Geometry check sheet. Reference: the model listing, model coordinates, mm. Round coordinates to 2 decimals unless told otherwise and drop trailing zeros. Use a Markdown table: item, result. Add a question column.
(1) Gauge pin test, flat ends, axial feed: P1, Ø17, axis at x = 3.27, z = 51.04, coming from the +Y side; P2, Ø4.5, axis at x = -8.04, z = -37.64, coming from the -Y side. Record the tip position at first contact, or that the pin passes through.
(2) Mould release check, pull along X, two halves, no side actions. Record for faces 1 (the face through (-9, 2, 71.041)), 2 (the face through (-8.64, 1.98, 37.82)), 3 (the face through (21.272, 2, 2)): released by +X, released by -X, zero draft, split by the parting line, or undercut.
(3) Section check A-A on y = 1.75. Give the number of separate pieces and of enclosed holes in the cut face, then the cut area to 3 significant figures.
(4) Thickness scan on line 1 along X through (y, z) = (3.25, -49); line 2 along X through (y, z) = (2.55, 38); line 3 along Z through (x, y) = (-2.5, 0.4). Record the ranges inside material, lowest first. Write a range as [from, to].
```python
from build123d import *

# Parameters (mm, degrees)
CROQUIS1_W              = 60
CROQUIS1_H              = 140
CROQUIS1_R              = 2
CROQUIS1_R_2            = 5
CROQUIS1_R_3            = 10.5
CROQUIS1_R_4            = 1.5
SALIENTE_EXTRUIR1_DEPTH = 4
CHAFL_N1_SIZE           = 0.5


with BuildPart() as part:
    # Croquis1 → Saliente-Extruir1 (new body)
    with BuildSketch(Plane(origin=(0, 0, 0), x_dir=(1, 0, 0), z_dir=(0, 1, 0))):
        with Locations((-8.728313692, -1.041413592)):
            Rectangle(CROQUIS1_W, CROQUIS1_H)
        with Locations(Location((3.271686308, 6.958586408, 0), (0, 0, 270))):
            Circle(CROQUIS1_R, mode=Mode.SUBTRACT)
        with Locations(Location((3.271686308, -9.041413592, 0), (0, 0, 270))):
            Circle(CROQUIS1_R, mode=Mode.SUBTRACT)
        with Locations(Location((14.585394807, 60.272294907, 0), (0, 0, 270))):
            Circle(CROQUIS1_R, mode=Mode.SUBTRACT)
        with Locations(Location((14.585394807, -39.727705093, 0), (0, 0, 270))):
            Circle(CROQUIS1_R, mode=Mode.SUBTRACT)
        with Locations(Location((-8.042022191, -39.727705093, 0), (0, 0, 90))):
            Circle(CROQUIS1_R, mode=Mode.SUBTRACT)
        with Locations(Location((-8.042022191, -62.355122091, 0), (0, 0, 270))):
            Circle(CROQUIS1_R, mode=Mode.SUBTRACT)
        with Locations(Location((3.271686308, -1.041413592, 0), (0, 0, 270))):
            Circle(CROQUIS1_R_2, mode=Mode.SUBTRACT)
        with Locations(Location((14.585394807, -62.355122091, 0), (0, 0, 90))):
            Circle(CROQUIS1_R, mode=Mode.SUBTRACT)
        with Locations(Location((3.271686308, -51.041413592, 0), (0, 0, 270))):
            Circle(CROQUIS1_R_3, mode=Mode.SUBTRACT)
        with Locations(Location((3.271686308, 48.958586408, 0), (0, 0, 270))):
            Circle(CROQUIS1_R_3, mode=Mode.SUBTRACT)
        with Locations(Location((-8.042022191, 60.272294907, 0), (0, 0, 90))):
            Circle(CROQUIS1_R, mode=Mode.SUBTRACT)
        with Locations(Location((14.585394807, 37.644877909, 0), (0, 0, 90))):
            Circle(CROQUIS1_R, mode=Mode.SUBTRACT)
        with Locations(Location((-8.042022191, 37.644877909, 0), (0, 0, 270))):
            Circle(CROQUIS1_R, mode=Mode.SUBTRACT)
        with Locations(Location((-21.728313692, -51.041413592, 0), (0, 0, 270))):
            Circle(CROQUIS1_R_4, mode=Mode.SUBTRACT)
        with Locations(Location((-33.728313692, -51.041413592, 0), (0, 0, 270))):
            Circle(CROQUIS1_R_4, mode=Mode.SUBTRACT)
        with Locations(Location((-21.728313692, 48.958586408, 0), (0, 0, 90))):
            Circle(CROQUIS1_R_4, mode=Mode.SUBTRACT)
        with Locations(Location((-33.728313692, 48.958586408, 0), (0, 0, 90))):
            Circle(CROQUIS1_R_4, mode=Mode.SUBTRACT)
    extrude(amount=SALIENTE_EXTRUIR1_DEPTH)

    # Chaflán1
    chafl_n1_edges = [part.edges().sort_by_distance(p)[0] for p in [
        (21.271686308, 4, 1.041413592),
        (3.271686308, 0, -8.958586408),
        (3.271686308, 4, -8.958586408),
        (-8.728313692, 4, -68.958586408),
        (3.271686308, 0, 7.041413592),
        (3.271686308, 4, 7.041413592),
        (14.585394807, 0, 37.727705093),
        (14.585394807, 4, 37.727705093),
        (-8.042022191, 0, 41.727705093),
        (-8.042022191, 4, 41.727705093),
        (3.271686308, 0, -3.958586408),
        (3.271686308, 4, -3.958586408),
        (-8.042022191, 0, 60.355122091),
        (-8.042022191, 4, 60.355122091),
        (3.271686308, 0, 40.541413592),
        (3.271686308, 4, 40.541413592),
        (3.271686308, 0, -59.458586408),
        (3.271686308, 4, -59.458586408),
        (-38.728313692, 4, 1.041413592),
        (14.585394807, 0, 64.355122091),
        (14.585394807, 4, 64.355122091),
        (-8.728313692, 0, -68.958586408),
        (14.585394807, 0, -62.272294907),
        (14.585394807, 4, -62.272294907),
        (21.271686308, 0, 1.041413592),
        (-8.042022191, 0, -58.272294907),
        (-8.042022191, 4, -58.272294907),
        (-8.728313692, 0, 71.041413592),
        (14.585394807, 0, -35.644877909),
        (14.585394807, 4, -35.644877909),
        (-38.728313692, 0, 1.041413592),
        (-8.042022191, 0, -39.644877909),
        (-8.042022191, 4, -39.644877909),
        (-21.728313692, 0, 49.541413592),
        (-21.728313692, 4, 49.541413592),
        (-33.728313692, 0, 49.541413592),
        (-33.728313692, 4, 49.541413592),
        (-21.728313692, 0, -47.458586408),
        (-21.728313692, 4, -47.458586408),
        (-8.728313692, 4, 71.041413592),
        (-33.728313692, 0, -47.458586408),
        (-33.728313692, 4, -47.458586408),
        (-38.728313692, 2, -68.958586408),
        (21.271686308, 2, -68.958586408),
        (21.271686308, 2, 71.041413592),
        (-38.728313692, 2, 71.041413592),
    ]]
    chamfer(chafl_n1_edges, length=CHAFL_N1_SIZE - 0.0001)  # a hair under: the kernel refuses the full size


solid = part.part
```
Check sheet entries:
| question | item | result |
|---|---|---|
| 1 | P1 | passes through |
| 1 | P2 | stops at y = 0.24 |
| 2 | face 1 | zero draft |
| 2 | face 2 | undercut |
| 2 | face 3 | released by +X |
| 3 | separate pieces | 1 |
| 3 | enclosed holes | 17 |
| 3 | area | 7,470 mm2 |
| 4 | line 1 | x = [-38.73, -35.23], [-32.23, -23.23], [-20.23, -7.23], [13.77, 21.27] |
| 4 | line 2 | x = [-38.73, -9.05], [-7.03, 13.58], [15.59, 21.27] |
| 4 | line 3 | z = [-68.86, -57.85], [-40.07, 42.15], [59.93, 70.94] |
